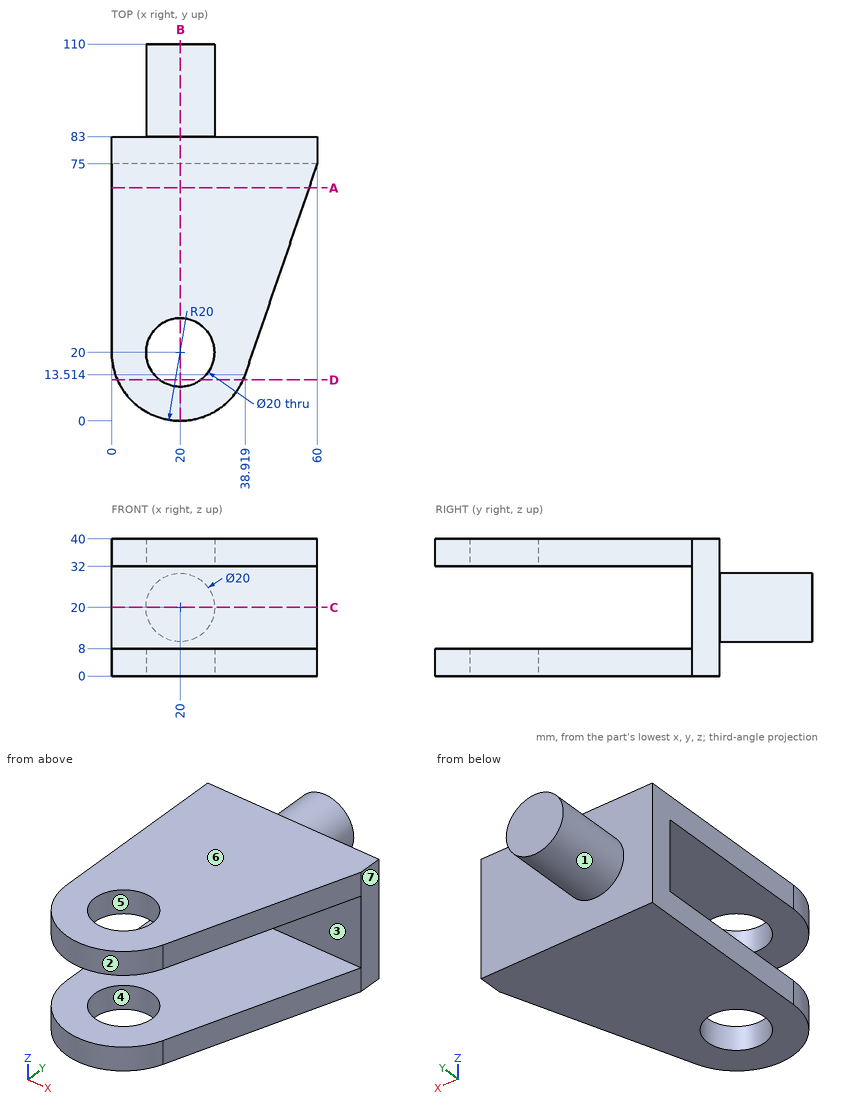
Study the drawing (mm; zero at the part's minimum x, y, z) and answer. A direction names the side the tool comes from. Give positions to 0.01 mm unless a question says otherwise; leave off trailing zeros. Order: outer loops, then holes, each group sorted by start corner. A loop starts at its lowest first (then second) coordinate and runs counter-clockwise, first axis right, second up.
1) Determine the mould class of the marked faces 4, 5, 6 and 7 for opening direction X: pulls with the +X half, pulls with the -X half, needs draft (parallel to the pull), parting line crosses it, or undercut.
Reported:
face 4: undercut
face 5: undercut
face 6: needs draft
face 7: pulls with the +X half
2) For the marked faces 1, 2 and 3, determine the directions among +Z, -Z, +X, -X, +Y, -Y from which every point of the face is accessible in a straight line to the end or side of a thin tool.
Reported:
face 1: +Y
face 2: +Z, -Z, -Y
face 3: +X, -X, -Y
3) Find section A-A on y = 68. Write down the section's boundary in (x, z).
Reported:
outline: (0, 0) - (57.6, 0) - (57.6, 8) - (0, 8) - close; (0, 32) - (57.6, 32) - (57.6, 40) - (0, 40) - close
4) Find section C-C on z = 20. Write down the section's boundary in (x, y), then the cut area to 3 significant figures.
Reported:
outline: (0, 75) - (60, 75) - (60, 83) - (30, 83) - (30, 110) - (10, 110) - (10, 83) - (0, 83) - close
area: 1,020 mm2
5) Consider line 1 along Y through (x, z) = (20, 5.5); line 2 along Z through (x, y) = (32, 67.5); line 3 along Y through (x, z) = (27, 15.5). Determine where each line is inside the solid, lowest interval first.
Reported:
line 1: y = 0 to 10, 30 to 83
line 2: z = 0 to 8, 32 to 40
line 3: y = 75 to 110
6) Given P1, Ø6, axis at y = 88.5, z = 16.5, coming from the +X side; P2, Ø12, axis at x = 25.5, z = 20.5, coming from the -Y side; P3, Ø2, axis at x = 25, z = 4.5, coming from the -Y side, each flat-ended and moving along its own axis, determine where each tip first touches the part or whether it passes through.
Reported:
P1: stops at x = 29.99
P2: stops at y = 75
P3: stops at y = 0.4
7) Find section B-B on x = 20. Write down the section's boundary in (y, z).
Reported:
outline: (0, 0) - (10, 0) - (10, 8) - (0, 8) - close; (0, 32) - (10, 32) - (10, 40) - (0, 40) - close; (30, 0) - (83, 0) - (83, 10) - (110, 10) - (110, 30) - (83, 30) - (83, 40) - (30, 40) - (30, 32) - (75, 32) - (75, 8) - (30, 8) - close
8) Find section D-D on y = 12. Write down the section's boundary in (x, z).
Reported:
outline: (1.67, 0) - (14, 0) - (14, 8) - (1.67, 8) - close; (1.67, 32) - (14, 32) - (14, 40) - (1.67, 40) - close; (26, 0) - (38.33, 0) - (38.33, 8) - (26, 8) - close; (26, 32) - (38.33, 32) - (38.33, 40) - (26, 40) - close
